```python
from build123d import *

# Parameters (mm, degrees)
MAINPIECE_DEPTH       = 40
CHASSISHOLES_REACH    = 75.546
SKETCH2_R             = 1.75
DOME_REACH            = 75.546
WHEELMOTORGUIDE_REACH = 75.546
SKETCH4_R             = 1.6
FILLET1_R             = 0.7


with BuildPart() as part:
    # Sketch1 → MainPiece (new body)
    with BuildSketch(Plane(origin=(0, 0, 0), x_dir=(0, 0, -1), z_dir=(1, 0, 0))):
        with BuildLine():
            Line((0, 1.5), (0, 0))
            Line((0, 0), (34.963274192, 0))
            ThreePointArc((34.963274192, 0), (38.524777166, 1.475222834), (40, 5.036725808))
            Line((40, 5.036725808), (40, 47))
            Line((40, 47), (38.5, 47))
            Line((38.5, 47), (38.5, 1.5))
            Line((38.5, 1.5), (0, 1.5))
        make_face()
    extrude(amount=MAINPIECE_DEPTH)

    # Sketch2 → ChassisHoles (cut, up to next)
    with BuildSketch(Plane(origin=(0, 0, 0), x_dir=(-1, 0, 0), z_dir=(0, -1, 0)), mode=Mode.PRIVATE) as chassisholes_sk1:
        with Locations(Location((-5, 8, 0), (0, 0, 90))):
            Circle(SKETCH2_R)
    chassisholes_tool1 = extrude(chassisholes_sk1.sketch, amount=-CHASSISHOLES_REACH, mode=Mode.PRIVATE) & part.part
    # Sketch2 → ChassisHoles (cut, up to next)
    with BuildSketch(Plane(origin=(0, 0, 0), x_dir=(-1, 0, 0), z_dir=(0, -1, 0)), mode=Mode.PRIVATE) as chassisholes_sk2:
        with Locations(Location((-35, 8, 0), (0, 0, 90))):
            Circle(SKETCH2_R)
    chassisholes_tool2 = extrude(chassisholes_sk2.sketch, amount=-CHASSISHOLES_REACH, mode=Mode.PRIVATE) & part.part
    # Sketch2 → ChassisHoles (cut, up to next)
    with BuildSketch(Plane(origin=(0, 0, 0), x_dir=(-1, 0, 0), z_dir=(0, -1, 0)), mode=Mode.PRIVATE) as chassisholes_sk3:
        with Locations(Location((-35, 32, 0), (0, 0, 90))):
            Circle(SKETCH2_R)
    chassisholes_tool3 = extrude(chassisholes_sk3.sketch, amount=-CHASSISHOLES_REACH, mode=Mode.PRIVATE) & part.part
    # Sketch2 → ChassisHoles (cut, up to next)
    with BuildSketch(Plane(origin=(0, 0, 0), x_dir=(-1, 0, 0), z_dir=(0, -1, 0)), mode=Mode.PRIVATE) as chassisholes_sk4:
        with Locations(Location((-5, 32, 0), (0, 0, 90))):
            Circle(SKETCH2_R)
    chassisholes_tool4 = extrude(chassisholes_sk4.sketch, amount=-CHASSISHOLES_REACH, mode=Mode.PRIVATE) & part.part
    add(chassisholes_tool1.solids().sort_by_distance((5, 0, -8))[0], mode=Mode.SUBTRACT)
    add(chassisholes_tool2.solids().sort_by_distance((35, 0, -8))[0], mode=Mode.SUBTRACT)
    add(chassisholes_tool3.solids().sort_by_distance((35, 0, -32))[0], mode=Mode.SUBTRACT)
    add(chassisholes_tool4.solids().sort_by_distance((5, 0, -32))[0], mode=Mode.SUBTRACT)

    # Sketch3 → Dome (cut, up to next)
    with BuildSketch(Plane(origin=(0, 0, -40), x_dir=(-1, 0, 0), z_dir=(0, 0, -1)), mode=Mode.PRIVATE) as dome_sk1:
        with BuildLine():
            Line((-40, 47), (-40, 27))
            ThreePointArc((-40, 27), (-34.142135624, 41.142135624), (-20, 47))
            Line((-20, 47), (-40, 47))
        make_face()
    dome_tool1 = extrude(dome_sk1.sketch, amount=-DOME_REACH, mode=Mode.PRIVATE) & part.part
    # Sketch3 → Dome (cut, up to next)
    with BuildSketch(Plane(origin=(0, 0, -40), x_dir=(-1, 0, 0), z_dir=(0, 0, -1)), mode=Mode.PRIVATE) as dome_sk2:
        with BuildLine():
            Line((0, 47), (-20, 47))
            ThreePointArc((-20, 47), (-5.857864376, 41.142135624), (0, 27))
            Line((0, 27), (0, 47))
        make_face()
    dome_tool2 = extrude(dome_sk2.sketch, amount=-DOME_REACH, mode=Mode.PRIVATE) & part.part
    add(dome_tool1.solids().sort_by_distance((35.532641, 42.532641, -40))[0], mode=Mode.SUBTRACT)
    add(dome_tool2.solids().sort_by_distance((4.467359, 42.532641, -40))[0], mode=Mode.SUBTRACT)

    # Sketch4 → WheelMotorGuide (cut, up to next)
    with BuildSketch(Plane(origin=(0, 0, -40), x_dir=(-1, 0, 0), z_dir=(0, 0, -1)), mode=Mode.PRIVATE) as wheelmotorguide_sk1:
        with Locations((-35.500160217, 27)):
            Circle(SKETCH4_R)
    wheelmotorguide_tool1 = extrude(wheelmotorguide_sk1.sketch, amount=-WHEELMOTORGUIDE_REACH, mode=Mode.PRIVATE) & part.part
    # Sketch4 → WheelMotorGuide (cut, up to next)
    with BuildSketch(Plane(origin=(0, 0, -40), x_dir=(-1, 0, 0), z_dir=(0, 0, -1)), mode=Mode.PRIVATE) as wheelmotorguide_sk2:
        with Locations((-27.750080108, 40.42353251)):
            Circle(SKETCH4_R)
    wheelmotorguide_tool2 = extrude(wheelmotorguide_sk2.sketch, amount=-WHEELMOTORGUIDE_REACH, mode=Mode.PRIVATE) & part.part
    # Sketch4 → WheelMotorGuide (cut, up to next)
    with BuildSketch(Plane(origin=(0, 0, -40), x_dir=(-1, 0, 0), z_dir=(0, 0, -1)), mode=Mode.PRIVATE) as wheelmotorguide_sk3:
        with Locations((-12.249919892, 40.42353251)):
            Circle(SKETCH4_R)
    wheelmotorguide_tool3 = extrude(wheelmotorguide_sk3.sketch, amount=-WHEELMOTORGUIDE_REACH, mode=Mode.PRIVATE) & part.part
    # Sketch4 → WheelMotorGuide (cut, up to next)
    with BuildSketch(Plane(origin=(0, 0, -40), x_dir=(-1, 0, 0), z_dir=(0, 0, -1)), mode=Mode.PRIVATE) as wheelmotorguide_sk4:
        with Locations((-4.499839783, 27)):
            Circle(SKETCH4_R)
    wheelmotorguide_tool4 = extrude(wheelmotorguide_sk4.sketch, amount=-WHEELMOTORGUIDE_REACH, mode=Mode.PRIVATE) & part.part
    # Sketch4 → WheelMotorGuide (cut, up to next)
    with BuildSketch(Plane(origin=(0, 0, -40), x_dir=(-1, 0, 0), z_dir=(0, 0, -1)), mode=Mode.PRIVATE) as wheelmotorguide_sk5:
        with Locations((-12.249919892, 13.57646749)):
            Circle(SKETCH4_R)
    wheelmotorguide_tool5 = extrude(wheelmotorguide_sk5.sketch, amount=-WHEELMOTORGUIDE_REACH, mode=Mode.PRIVATE) & part.part
    # Sketch4 → WheelMotorGuide (cut, up to next)
    with BuildSketch(Plane(origin=(0, 0, -40), x_dir=(-1, 0, 0), z_dir=(0, 0, -1)), mode=Mode.PRIVATE) as wheelmotorguide_sk6:
        with Locations((-27.750080108, 13.57646749)):
            Circle(SKETCH4_R)
    wheelmotorguide_tool6 = extrude(wheelmotorguide_sk6.sketch, amount=-WHEELMOTORGUIDE_REACH, mode=Mode.PRIVATE) & part.part
    # Sketch4 → WheelMotorGuide (cut, up to next)
    with BuildSketch(Plane(origin=(0, 0, -40), x_dir=(-1, 0, 0), z_dir=(0, 0, -1)), mode=Mode.PRIVATE) as wheelmotorguide_sk7:
        with BuildLine():
            Line((-26.5, 20), (-26.5, 34))
            ThreePointArc((-26.5, 34), (-20, 40.5), (-13.5, 34))
            Line((-13.5, 34), (-13.5, 20))
            ThreePointArc((-13.5, 20), (-20, 13.5), (-26.5, 20))
        make_face()
    wheelmotorguide_tool7 = extrude(wheelmotorguide_sk7.sketch, amount=-WHEELMOTORGUIDE_REACH, mode=Mode.PRIVATE) & part.part
    add(wheelmotorguide_tool1.solids().sort_by_distance((35.50016, 27, -40))[0], mode=Mode.SUBTRACT)
    add(wheelmotorguide_tool2.solids().sort_by_distance((27.75008, 40.423533, -40))[0], mode=Mode.SUBTRACT)
    add(wheelmotorguide_tool3.solids().sort_by_distance((12.24992, 40.423533, -40))[0], mode=Mode.SUBTRACT)
    add(wheelmotorguide_tool4.solids().sort_by_distance((4.49984, 27, -40))[0], mode=Mode.SUBTRACT)
    add(wheelmotorguide_tool5.solids().sort_by_distance((12.24992, 13.576467, -40))[0], mode=Mode.SUBTRACT)
    add(wheelmotorguide_tool6.solids().sort_by_distance((27.75008, 13.576467, -40))[0], mode=Mode.SUBTRACT)
    add(wheelmotorguide_tool7.solids().sort_by_distance((20, 27, -40))[0], mode=Mode.SUBTRACT)

    # Fillet1
    fillet1_edges = [part.edges().sort_by_distance(p)[0] for p in [
        (20, 1.5, -38.5),
        (40, 0.75, 0),
        (0, 0.75, 0),
    ]]
    fillet(fillet1_edges, radius=FILLET1_R)


solid = part.part
```
Build history of the part. All positions in model axes, mm. A direction names the side the tool comes from. Give positions to 0.01 mm unless a question says otherwise; leave off trailing zeros. Loops run counter-clockwise (first coordinate to the right, second up) from the corner with the lowest first, then second, coordinate; pieces in that order, holes last. Notation, with made-up numbers: (-20, -18) -> (6, -18) arc R29 cw to (6, 8) -> close; hole circle Ø9 at (80, 10.5). An arc over 180 degrees is marked (long way). One line per question, with ' | ' between items. Start each with the question number.
1) Cut at C-C (x = 35). Give the cut face in (y, z).
2) Cut at D-D (y = 10.5). Give the cut face in (x, z), plus the area to 3 significant figures.
3) Cut at B-B (y = 16). Give the cut face in (x, z).
4) 3-axis set-ups, long thin cutter, end or side, ignore diameter. For faces 1 (the flat face through (15, 15, -38.5)), 2 (the cylindrical face through (35.08, 0.74, -30.25)), 3 (the cylindrical face through (19.9, 13.5, -39.3)): which of +Z, -Z, +X, -X, +Y, -Y reach the whole face in a straight line?
5) Cut at A-A (z = -32). Give the cut face in (x, y), plus the area to 3 significant figures.
6) Two-plate mould, pull along X, no slides. Class faces 4 (the cylindrical face through (12.46, 42.01, -39.26)), 5 (the flat face through (11, 21, -40)), 6 (the cylindrical face through (5.08, 0.74, -30.25)), 7 (the flat face through (40, 1, -29)): released by +X, released by -X, zero draft, split by the parting line, or undercut.
7) Probe L1, parallel to X at y = 1, z = -8; L2, parallel to Z at x = 22, y = 12; L3, parallel to Y at x = 34.5, z = -22.5. List the from-to ranges inside material, lowest first.
8) Pin check, flat tips, straight feed: pin 1 (2.5 mm diameter, centred on x = 12.25, y = 13.58, fed in from +Z); pin 2 (3 mm diameter, centred on x = 23.5, z = -30, fed in from -Y); pin 3 (10 mm diameter, centred on x = 21, y = 38, fed in from +Z); pin 4 (6 mm diameter, centred on x = 13, z = -29.5, fed in from +Y). Stop position of each tip, or through.
Return value:
1) outline: (0, -34.96) arc R5.04 ccw to (5.04, -40) -> (25.48, -40) -> (25.48, -38.5) -> (2.2, -38.5) arc R0.7 cw to (1.5, -37.8) -> (1.5, -33.75) -> (0, -33.75) -> close; (0, -30.25) -> (1.5, -30.25) -> (1.5, -9.75) -> (0, -9.75) -> close; (0, -6.25) -> (1.5, -6.25) -> (1.5, 0) -> (0, 0) -> close; (28.52, -40) -> (40.23, -40) -> (40.23, -38.5) -> (28.52, -38.5) -> close
2) outline: (0, -40) -> (40, -40) -> (40, -38.5) -> (0, -38.5) -> close | area: 60.0 mm^2
3) outline: (0, -40) -> (14.88, -40) -> (14.88, -38.5) -> (0, -38.5) -> close; (25.12, -40) -> (40, -40) -> (40, -38.5) -> (25.12, -38.5) -> close
4) face 1: +Z, +X, -X, +Y | face 2: +Y, -Y | face 3: +Z, -Z
5) outline: (0, 0) -> (3.25, 0) -> (3.25, 1.5) -> (0, 1.5) -> close; (6.75, 0) -> (33.25, 0) -> (33.25, 1.5) -> (6.75, 1.5) -> close; (36.75, 0) -> (40, 0) -> (40, 1.5) -> (36.75, 1.5) -> close | area: 49.5 mm^2
6) face 4: undercut | face 5: zero draft | face 6: undercut | face 7: released by +X
7) L1: 0 to 3.25, 6.75 to 33.25, 36.75 to 40 | L2: -40 to -38.5 | L3: 0 to 1.5
8) pin 1: through | pin 2: y = 0 | pin 3: z = -38.5 | pin 4: y = 1.5
